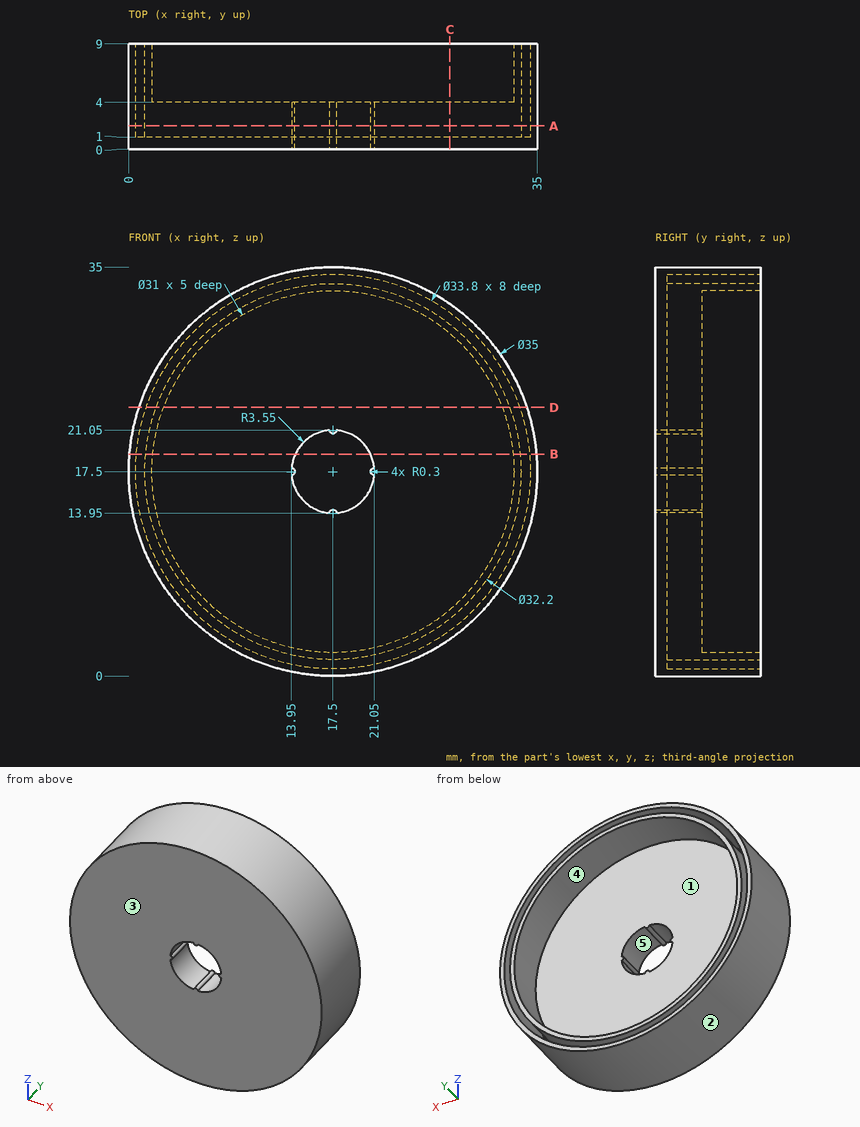
Input: dimensioned drawing with shaded views. Units: mm. Origin: part minimum x, y, z. A direction names the side the tool comes from. Round coordinates to 2 decimals unless told otherwise and drop trailing zeros. Loops run counter-clockwise (first coordinate to the right, second up) from the corner with the lowest first, then second, coordinate; pieces in that order, holes last. Notation, with made-up numbers: (39, 43) -> (73, 43) arc R18 ccw to (73, 58) -> close; hole circle Ø5 at (19.5, -3.5). An arc over 180 degrees is marked (long way). Answer as a JSON object with one key per item and string values. Group by question number.
Q1. Ray query, line 1 (Z direction, x = 17.5, y = 7.5); line 2 (X direction, y = 4.75, z = 17); line 3 (X direction, y = 3.5, z = 17.5). Return the intervals inside material, ascending. Write a range as from..to.
Q2. Contact query for flat-ended pins moving along their axis: P1, Ø10, axis at x = 17, z = 9.5, coming from the +Y side; P2, Ø1.5, axis at x = 8, y = 7.5, coming from the +Z side; P3, Ø5, axis at y = 6.5, z = 7.5, coming from the -X side. Output: stop coordinate, or through.
Q3. Section query C-C (x = 27.5). Output: boundary loops of the cut face in (y, z), plus the area to 3 significant figures.
Q4. Section query D-D (z = 23). Output: boundary loops of the cut face in (x, y), plus the area to 3 significant figures.
Q5. Section query B-B (z = 19). Output: boundary loops of the cut face in (x, y).
Q6. Mould query, pull axis X, two halves, no side actions, for the marked faces 1, 2 and 3. Classes: pulls with the +X half, pulls with the -X half, needs draft (parallel to the pull), parting line crosses it, or undercut.
Q7. Access query for the marked faces 4 and 5. Directions: +Z, -Z, +X, -X, +Y, -Y. A direction counts if a zero-diameter tool reaches every point of the face in a straight line with its end or side. Return the directions, or none.
Q8. Section query A-A (y = 2). Output: boundary loops of the cut face in (x, z).
Completed:
{
 "1": {"line 1": "0..0.6, 1.4..2, 33..33.6, 34.4..35", "line 2": "0.01..0.61, 1.41..2.01, 32.99..33.59, 34.39..34.99", "line 3": "0..0.6, 1.4..14.25, 20.75..33.6, 34.4..35"},
 "2": {"P1": "y = 4", "P2": "z = 32.66", "P3": "x = 1.69"},
 "3": {"outline": "(0, 3.14) -> (9, 3.14) -> (9, 3.88) -> (1, 3.88) -> (1, 4.88) -> (9, 4.88) -> (9, 5.66) -> (4, 5.66) -> (4, 29.34) -> (9, 29.34) -> (9, 30.12) -> (1, 30.12) -> (1, 31.12) -> (9, 31.12) -> (9, 31.86) -> (0, 31.86) -> close", "area": "124 mm²"},
 "4": {"outline": "(0.89, 0) -> (34.11, 0) -> (34.11, 9) -> (33.48, 9) -> (33.48, 1) -> (32.63, 1) -> (32.63, 9) -> (31.99, 9) -> (31.99, 4) -> (3.01, 4) -> (3.01, 9) -> (2.37, 9) -> (2.37, 1) -> (1.52, 1) -> (1.52, 9) -> (0.89, 9) -> close", "area": "141 mm²"},
 "5": {"outline": "(0.06, 0) -> (14.28, 0) -> (14.28, 4) -> (2.07, 4) -> (2.07, 9) -> (1.47, 9) -> (1.47, 1) -> (0.67, 1) -> (0.67, 9) -> (0.06, 9) -> close; (20.72, 0) -> (34.94, 0) -> (34.94, 9) -> (34.33, 9) -> (34.33, 1) -> (33.53, 1) -> (33.53, 9) -> (32.93, 9) -> (32.93, 4) -> (20.72, 4) -> close"},
 "6": {"face 1": "undercut", "face 2": "parting line crosses it", "face 3": "needs draft"},
 "7": {"face 4": "+Y", "face 5": "+Y, -Y"},
 "8": {"outline": "circle Ø35 at (17.5, 17.5); circle Ø32.2 at (17.5, 17.5); hole circle Ø33.8 at (17.5, 17.5); hole (13.96, 17.2) arc R3.55 ccw to (17.2, 13.96) arc R0.3 cw to (17.8, 13.96) arc R3.55 ccw to (21.04, 17.2) arc R0.3 cw to (21.04, 17.8) arc R3.55 ccw to (17.8, 21.04) arc R0.3 cw to (17.2, 21.04) arc R3.55 ccw to (13.96, 17.8) arc R0.3 cw to start"}
}
